```python
from build123d import *

# Parameters (mm, degrees)
BOSS_EXTRUDE1_DEPTH = 2.7
SKETCH3_R           = 2.5
CUT_EXTRUDE1_DEPTH  = 0.3
SKETCH4_R           = 2
BOSS_EXTRUDE2_DEPTH = 16.28
BOSS_EXTRUDE3_DEPTH = 1
SKETCH7_R           = 4.35
BOSS_EXTRUDE4_DEPTH = 0.65
SKETCH8_W           = 1
SKETCH8_H           = 1.6
SKETCH8_H_2         = 1
SKETCH8_W_2         = 1.6
CUT_EXTRUDE2_DEPTH  = 2
FILLET1_R           = 1
CHAMFER1_SIZE       = 0.2


with BuildPart() as part:
    # Sketch2 → Boss-Extrude1 (new body)
    with BuildSketch(Plane(origin=(0, 0, 0), x_dir=(1, 0, 0), z_dir=(0, 1, 0))):
        Polygon((0, -3.983716857), (3.45, -1.991858429), (3.45, 1.991858429), (0, 3.983716857), (-3.45, 1.991858429), (-3.45, -1.991858429), align=None)
    extrude(amount=BOSS_EXTRUDE1_DEPTH)

    # Sketch3 → Cut-Extrude1 (cut)
    with BuildSketch(Plane(origin=(0, 2.7, 0), x_dir=(1, 0, 0), z_dir=(0, 1, 0))):
        with Locations(Location((0, 0, 0), (0, 0, 270))):
            Circle(SKETCH3_R)
    extrude(amount=-CUT_EXTRUDE1_DEPTH, mode=Mode.SUBTRACT)

    # Sketch4 → Boss-Extrude2 (add)
    with BuildSketch(Plane.XZ):
        with Locations(Location((0, 0, 0), (0, 0, 270))):
            Circle(SKETCH4_R)
    extrude(amount=BOSS_EXTRUDE2_DEPTH)

    # Sketch5 → Boss-Extrude3 (add)
    with BuildSketch(Plane.XZ):
        with BuildLine():
            Line((0, 2.15), (0, 3.15))
            ThreePointArc((0, 3.15), (-0.250796162, -3.140000205), (0.5, 3.110064308))
            Line((0.5, 3.110064308), (0.5, 2.091052367))
            ThreePointArc((0.5, 2.091052367), (-0.251731416, -2.135212236), (0, 2.15))
        make_face()
    extrude(amount=BOSS_EXTRUDE3_DEPTH)

    # Sketch7 → Boss-Extrude4 (add)
    with BuildSketch(Plane.XZ.offset(1)):
        with Locations(Location((0, 0, 0), (0, 0, 270))):
            Circle(SKETCH7_R)
    extrude(amount=BOSS_EXTRUDE4_DEPTH)

    # Sketch8 → Cut-Extrude2 (cut)
    with BuildSketch(Plane(origin=(0, 2.4, 0), x_dir=(1, 0, 0), z_dir=(0, 1, 0))):
        with Locations((0, 1.3)):
            Rectangle(SKETCH8_W, SKETCH8_H)
        Rectangle(SKETCH8_W, SKETCH8_H_2)
        with Locations((-1.3, 0)):
            Rectangle(SKETCH8_W_2, SKETCH8_H_2)
        with Locations((0, -1.3)):
            Rectangle(SKETCH8_W, SKETCH8_H)
        with Locations((1.3, 0)):
            Rectangle(SKETCH8_W_2, SKETCH8_H_2)
    extrude(amount=-CUT_EXTRUDE2_DEPTH, mode=Mode.SUBTRACT)

    # Fillet1
    fillet1_edges = [part.edges().sort_by_distance(p)[0] for p in [
        (-0.5, 1.4, -0.5),
        (0.5, 1.4, -0.5),
        (0.5, 1.4, 0.5),
        (-0.5, 1.4, 0.5),
    ]]
    fillet(fillet1_edges, radius=FILLET1_R)

    # Sketch9 → Cut-Revolve1 (revolve, cut)
    with BuildSketch(Plane(origin=(0, 0, 0), x_dir=(0, 0, -1), z_dir=(1, 0, 0))):
        Polygon((-3.983716857, 2.7), (-3.483716857, 2.7), (-3.983716857, 2.2), align=None)
        Polygon((-3.983716857, 0.5), (-3.983716857, 0), (-3.483716857, 0), align=None)
    revolve(axis=Axis((0, 0, 0), (0, -1, 0)), mode=Mode.SUBTRACT)

    # Chamfer1
    chamfer1_edges = [part.edges().sort_by_distance(p)[0] for p in [
        (0, -16.28, 2),
    ]]
    chamfer(chamfer1_edges, length=CHAMFER1_SIZE)


solid = part.part
```
For this review, take the finished solid that the model builds, in its own axes (mm). A direction names the side the tool comes from. Round coordinates to 2 decimals unless told otherwise and drop trailing zeros. Loops run counter-clockwise (first coordinate to the right, second up) from the corner with the lowest first, then second, coordinate; pieces in that order, holes last.
(1) We need section C-C (y = -3.75). Give the boundary of the cut face in (x, z).
Returned:
outline: circle Ø4 at (0, 0)
(2) Clearance check with flat-ended pins moving along their axes: P1, Ø1.4, axis at y = 1, z = -1, coming from the -X side; P2, Ø5, axis at x = 1.5, y = -13.5, coming from the -Z side; P3, Ø1, axis at x = -1.5, y = -9, coming from the -Z side. State where each tip first meets the part, or that it passes through.
Returned:
P1: stops at x = -3.45
P2: stops at z = -2
P3: stops at z = -1.73
(3) Tool access review of faces 4 (the flat face through (-2, -1.65, -1)), 5 (the flat face through (-3, -1, -2)), 6 (the flat face through (0, 1, 2.1)): name each direction out of +Z, -Z, +X, -X, +Y, -Y from which nothing blocks a thin tool from reaching the whole face with its end or side.
Returned:
face 4: -Y
face 5: none
face 6: +Y
(4) Wall thickness on line 1 along X through (y, z) = (2.65, 0); line 2 along Y through (x, z) = (1, 1); line 3 along Y through (x, z) = (-1.5, 3): over which ranges is each line inside the solid? List them lowest first.
Returned:
line 1: x = -3.45 to -2.5, 2.5 to 3.45
line 2: y = -16.28 to 2.4
line 3: y = -1.65 to -1, 0 to 2.7
(5) We need section B-B (y = 1). Give the boundary of the cut face in (x, z), plus the area to 3 significant figures.
Returned:
outline: (-3.45, -1.99) - (0, -3.98) - (3.45, -1.99) - (3.45, 1.99) - (0, 3.98) - (-3.45, 1.99) - close; hole (-2.1, -0.5) - (-1.5, -0.5) arc R1 cw to (-0.5, -1.5) - (-0.5, -2.1) - (0.5, -2.1) - (0.5, -1.5) arc R1 cw to (1.5, -0.5) - (2.1, -0.5) - (2.1, 0.5) - (1.5, 0.5) arc R1 cw to (0.5, 1.5) - (0.5, 2.1) - (-0.5, 2.1) - (-0.5, 1.5) arc R1 cw to (-1.5, 0.5) - (-2.1, 0.5) - close
area: 33.0 mm2
(6) We need section A-A (z = 0). State how many separate pieces and enclosed holes the cut face has, plus the area to 3 significant figures.
Returned:
separate pieces: 1
enclosed holes: 2
area: 78.9 mm2
(7) Mouldability with a two-part tool opening along Y and no side actions: class faces 1 (the conical face through (-3.15, 2.558, -1.796)), 2 (the flat face through (-2.1, 1, 0)), 3 (the flat face through (0, -0.5, 2.6)) as released by +Y, released by -Y, zero draft, split by the parting line, or undercut.
Returned:
face 1: released by +Y
face 2: zero draft
face 3: undercut
